from build123d import *

# Parameters (mm, degrees)
EXTRUDE_THIN1_DEPTH = 24


with BuildPart() as part:
    # Sketch1 → Extrude-Thin1 (new body, symmetric)
    with BuildSketch(Plane.XY):
        Polygon((-81.476659403, -37.476659403), (-44, 0), (44, 0), (81.476659403, -37.476659403), (75.112698372, -43.840620434), (40.272077939, -9), (-40.272077939, -9), (-75.112698372, -43.840620434), align=None)
    extrude(amount=EXTRUDE_THIN1_DEPTH, both=True)


solid = part.part
Input: part model. Units: mm. Frame: model coordinates. A direction names the side the tool comes from. Give positions to 0.01 mm unless a question says otherwise; leave off trailing zeros. Order: outer loops, then holes, each group sorted by start corner. A loop starts at its lowest first (then second) coordinate and runs counter-clockwise, first axis right, second up. Notation, with made-up numbers: (71.25, 85) - (99.25, 85) arc R7 cw to (99.25, 95) - close; hole circle Ø9 at (10, 38.25). An arc over 180 degrees is marked (long way). Write each question's results on one line, items separated by ' | '.
Item 1: Section B-B (y = -10.5). Return loops of the section in (x, z).
A:
outline: (-54.5, -24) - (-41.77, -24) - (-41.77, 24) - (-54.5, 24) - close; (41.77, -24) - (54.5, -24) - (54.5, 24) - (41.77, 24) - close
Item 2: Contact query for flat-ended pins moving along their axis: pin 1 Ø4 at (y, z) = (-13.5, 15.5) entering from -X; pin 2 Ø4 at (x, z) = (48, 7.5) entering from -Y; pin 3 Ø1 at (x, z) = (57.5, 11.5) entering from +Y. Output: stop coordinate, or through.
A:
pin 1: stops at x = -59.5 | pin 2: stops at y = -18.73 | pin 3: stops at y = -13
Item 3: Material intervals for line 1 along X through (y, z) = (-14, 16.5); line 2 along Y through (x, z) = (-31, 9); line 3 along X through (y, z) = (-36, -21), sorted ascending.
A:
line 1: x = -58 to -45.27, 45.27 to 58 | line 2: y = -9 to 0 | line 3: x = -80 to -67.27, 67.27 to 80
Item 4: Draft query along X for faces 1 (the flat face through (0.4, -8.8, 24)), 2 (the flat face through (1, -9, 0)), 3 (the flat face through (-57.45, -26.18, 0.34)), 4 (the flat face through (78.339, -40.614, 0.336)). Return one class per face: released by +X, released by -X, zero draft, split by the parting line, or undercut.
A:
face 1: zero draft | face 2: undercut | face 3: undercut | face 4: released by +X
Item 5: Section D-D (x = -58). Return loops of the section in (y, z), and give its area (3 significant figures).
A:
outline: (-26.73, -24) - (-14, -24) - (-14, 24) - (-26.73, 24) - close | area: 611 mm^2
Item 6: Access query for faces 5 (the flat face through (0.4, -8.8, -24)), 6 (the flat face through (57.936, -26.664, 0.336)). Directions: +Z, -Z, +X, -X, +Y, -Y. A direction counts if a zero-diameter tool reaches every point of the face in a straight line with its end or side. Return the directions, or none.
A:
face 5: -Z, +X, -X, +Y, -Y | face 6: +Z, -Z, -Y
Item 7: Section A-A (z = 12). Return loops of the section in (x, y), and give its area (3 significant figures).
A:
outline: (-81.48, -37.48) - (-75.11, -43.84) - (-40.27, -9) - (40.27, -9) - (75.11, -43.84) - (81.48, -37.48) - (44, 0) - (-44, 0) - close | area: 1,680 mm^2
Item 8: Section C-C (x = -5.5). Return loops of the section in (y, z).
A:
outline: (-9, -24) - (0, -24) - (0, 24) - (-9, 24) - close
